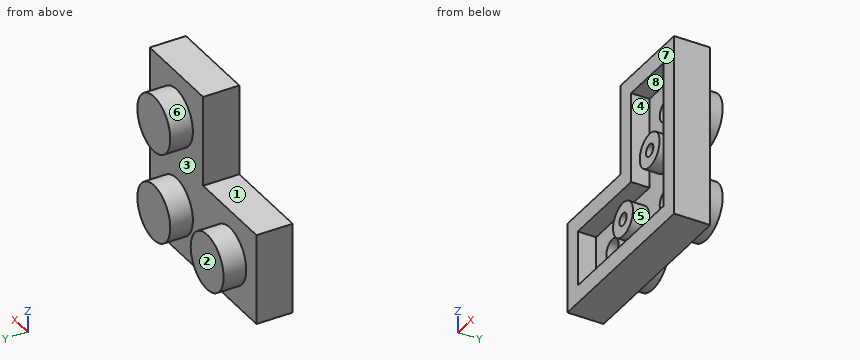
```python
from build123d import *

# Parameters (mm, degrees)
BOSS_EXTRUDE1_DEPTH = 3.15
SKETCH2_R           = 2.45
BOSS_EXTRUDE2_DEPTH = 1.97
SHELL1_T            = -1.55
SKETCH3_R           = 1.48
SKETCH3_R_2         = 0.54
BOSS_EXTRUDE3_DEPTH = 1.4


with BuildPart() as part:
    # Sketch1 → Boss-Extrude1 (new body)
    with BuildSketch(Plane(origin=(0, 0, 0), x_dir=(1, 0, 0), z_dir=(0, 1, 0))):
        Polygon((0, 0), (0, -7.945), (7.945, -7.945), (7.945, 7.945), (-7.945, 7.945), (-7.945, 0), align=None)
    extrude(amount=-BOSS_EXTRUDE1_DEPTH)

    # Sketch2 → Boss-Extrude2 (add)
    with BuildSketch(Plane(origin=(0, 0, 0), x_dir=(1, 0, 0), z_dir=(0, 1, 0))):
        with Locations(Location((3.9725, 3.9725, 0), (0, 0, 90))):
            Circle(SKETCH2_R)
        with Locations(Location((3.9725, -3.9725, 0), (0, 0, 90))):
            Circle(SKETCH2_R)
        with Locations(Location((-3.9725, 3.9725, 0), (0, 0, 90))):
            Circle(SKETCH2_R)
    extrude(amount=BOSS_EXTRUDE2_DEPTH)

    # Shell1
    shell1_openings = [part.faces().sort_by_distance(p)[0] for p in [
        (1.324166667, -3.15, -1.324166667),
    ]]
    offset(amount=SHELL1_T, openings=shell1_openings, kind=Kind.INTERSECTION)

    # Sketch3 → Boss-Extrude3 (add)
    # profile 1 of 2: a face of its own
    with BuildSketch(Plane.XZ.offset(1.55)):
        with Locations(Location((0, -3.975, 0), (0, 0, 270))):
            Circle(SKETCH3_R)
        with Locations(Location((0, -3.975, 0), (0, 0, 270))):
            Circle(SKETCH3_R_2, mode=Mode.SUBTRACT)
    # profile 2 of 2: a face of its own
    with BuildSketch(Plane.XZ.offset(1.55)):
        with Locations(Location((3.97, 0, 0), (0, 0, 270))):
            Circle(SKETCH3_R)
        with Locations(Location((3.97, 0, 0), (0, 0, 270))):
            Circle(SKETCH3_R_2, mode=Mode.SUBTRACT)
    extrude(amount=BOSS_EXTRUDE3_DEPTH)


solid = part.part
```
Check sheet for the modelled part. Datum: model origin and axes. Units: mm. Face numbers are marked on the shaded views. A direction names the side the tool comes from. Round coordinates to 2 decimals unless told otherwise and drop trailing zeros. Loops run counter-clockwise (first coordinate to the right, second up) from the corner with the lowest first, then second, coordinate; pieces in that order, holes last. Notation, with made-up numbers: M 33,59 L 67,59 A21 ccw 67,83 Z; hole C 27.5,88.5 d10. An arc over 180 degrees is marked long. Answer as a JSON object with one key per item and string values.
1. Section check A-A (y = -1.9). Record the boundary of the cut face in (x, z) (3 decimals), plus the area to 3 significant figures.
Reply:
{"outline": "M -7.945,-7.945 L 7.945,-7.945 L 7.945,7.945 L 0,7.945 L 0,0 L -7.945,0 Z; C 0,-3.975 d2.96; C 3.97,0 d2.96; hole M -6.395,-6.395 L 6.395,-6.395 L 6.395,6.395 L 1.55,6.395 L 1.55,-1.55 L -6.395,-1.55 Z; hole C 0,-3.975 d1.08; hole C 3.97,0 d1.08", "area": "101 mm²"}
2. Gauge pin test, flat ends, axial feed: P1, Ø1.6, axis at x = -3.97, z = -3.97, coming from the -Y side; P2, Ø1.5, axis at y = -2, z = 5.5, coming from the -X side; P3, Ø0.9, axis at x = 4, z = 0, coming from the -Y side. Record the tip position at first contact, or that the pin passes through.
Reply:
{"P1": "stops at y = 0.42", "P2": "stops at x = 0", "P3": "stops at y = -1.55"}
3. Access from +Z, -Z, +X, -X, +Y, -Y to the whole of each face (thin tool, end or side, straight path). Record for the marked faces 1, 2, 3 and 4.
Reply:
{"face 1": "+Z, -X, +Y, -Y", "face 2": "+Z, -Z, +X, -X, +Y", "face 3": "+Y", "face 4": "-Y"}
4. Scan lines: line 1 (Z direction, x = 4, y = -0.05) (3 decimals); line 2 (Z direction, x = 4.75, y = -0.95) (3 decimals); line 3 (X direction, y = -1.8, z = 0.25) (3 decimals). Record each from-to range of solid material in increasing order.
Reply:
{"line 1": "z = -7.945 to -4.872, -3.073 to 3.073, 4.872 to 7.945", "line 2": "z = -7.945 to -4.426, -3.519 to 3.519, 4.426 to 7.945", "line 3": "x = 0 to 1.55, 2.511 to 3.491, 4.449 to 5.429, 6.395 to 7.945"}
5. Section check C-C (x = -7). Record the boundary of the cut face in (y, z) (3 decimals).
Reply:
{"outline": "M -3.15,-7.945 L 0,-7.945 L 0,0 L -3.15,0 Z"}
6. Section check B-B (z = 5.5). Record the boundary of the cut face in (x, y) (3 decimals), plus the area to 3 significant figures.
Reply:
{"outline": "M 0,-3.15 L 1.55,-3.15 L 1.55,-1.55 L 6.395,-1.55 L 6.395,-3.15 L 7.945,-3.15 L 7.945,0 L 5.888,0 L 5.888,1.97 L 2.057,1.97 L 2.057,0 L 0,0 Z", "area": "24.8 mm²"}
7. Mould release check, pull along X, two halves, no side actions. Record for the marked faces 5, 6, 7 and 8: pulls with the +X half, pulls with the -X half, needs draft (parallel to the pull), parting line crosses it, or undercut.
Reply:
{"face 5": "undercut", "face 6": "parting line crosses it", "face 7": "needs draft", "face 8": "undercut"}
8. Section check D-D (y = 0.65). Record the boundary of the cut face in (x, z), plus the area to 3 significant figures.
Reply:
{"outline": "C -3.97,-3.97 d4.9; C 3.97,-3.97 d4.9; C 3.97,3.97 d4.9", "area": "56.6 mm²"}
